from build123d import *

# Parameters (mm, degrees)
SKETCH_1_W          = 66
SKETCH_1_H          = 80.5
EXTRUDE_1_DEPTH     = 5
SKETCH_2_R          = 2
CUT_EXTRUDE_1_DEPTH = 53.288263501
SKETCH_3_R          = 2.1
CUT_EXTRUDE_2_DEPTH = 10
FILLET_1_R          = 15


with BuildPart() as part:
    # 草图1 → 凸台-拉伸1 (new body)
    with BuildSketch(Plane.XY):
        Rectangle(SKETCH_1_W, SKETCH_1_H)
    extrude(amount=EXTRUDE_1_DEPTH)

    # 草图2 → 切除-拉伸1 (cut, through all)
    with BuildSketch(Plane.XY.offset(5)):
        with Locations((-26, 35.25)):
            Circle(SKETCH_2_R)
        with Locations((26, 35.25)):
            Circle(SKETCH_2_R)
        with Locations((26, 25.25)):
            Circle(SKETCH_2_R)
        with Locations((-26, 25.25)):
            Circle(SKETCH_2_R)
    extrude(amount=-CUT_EXTRUDE_1_DEPTH, mode=Mode.SUBTRACT)

    # 草图3 → 切除-拉伸2 (cut)
    with BuildSketch(Plane.XY.offset(5)):
        with Locations((-11, 0.25)):
            Circle(SKETCH_3_R)
        with Locations((11, 0.25)):
            Circle(SKETCH_3_R)
        with Locations((11, -19.75)):
            Circle(SKETCH_3_R)
        with Locations((-11, -19.75)):
            Circle(SKETCH_3_R)
    extrude(amount=-CUT_EXTRUDE_2_DEPTH, mode=Mode.SUBTRACT)

    # 圆角1
    fillet_1_edges = [part.edges().sort_by_distance(p)[0] for p in [
        (33, -40.25, 2.5),
        (-33, -40.25, 2.5),
    ]]
    fillet(fillet_1_edges, radius=FILLET_1_R)


solid = part.part
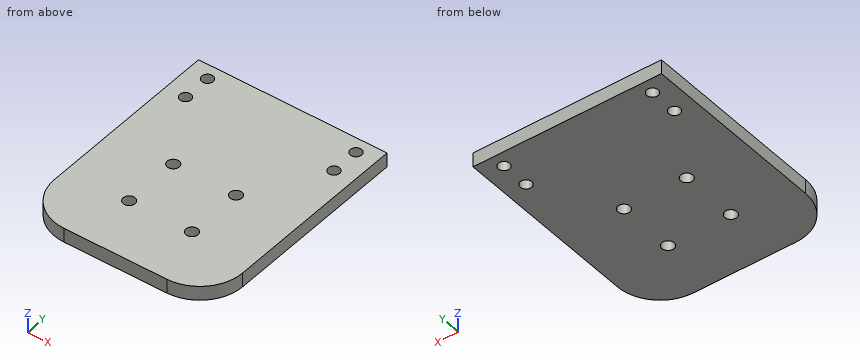
The model under review builds one solid part; all positions refer to its coordinate system, in mm. Round coordinates to 2 decimals unless told otherwise and drop trailing zeros. Write each loop counter-clockwise with the first axis right and the second up, starting at its lowest first coordinate (ties: lowest second). Pieces come first, ordered by that corner, then holes. Notation, with made-up numbers: M 4,82 L 25,82 A17 cw 25,87 Z; hole C 25,-0.75 d2. An arc over 180 degrees is marked long. Answer as CSV lines item,"result". Start each with the question number.
Q1. Consider section A-A, the plane y = 35.25. Give the boundary of the cut face in (x, z), then the cut area to 3 significant figures.
Q2. Consider section B-B, the plane x = -11. Give the boundary of the cut face in (y, z), then the cut area to 4 significant figures.
Q3. Consider section C-C, the plane z = 1.4. State how many separate pieces and enclosed holes the cut face has, then the cut area to 3 significant figures.
Q4. Wall thickness on line 1 along Y through (x, z) = (11, 2.45); line 2 along Y through (x, z) = (26, 1.35); line 3 along Y through (x, z) = (18.5, 1.75): over which ranges is each line inside the solid? List them lowest first.
Q5. Clearance check with a flat-ended pin moving along its axis: P1, Ø2.5, axis at x = 26, y = 25.25, coming from the -Z side. State where the tip first meets the part, or that it passes through.
Result set:
1,outline,"M -33,0 L -28,0 L -28,5 L -33,5 Z; M -24,0 L 24,0 L 24,5 L -24,5 Z; M 28,0 L 33,0 L 33,5 L 28,5 Z"
1,area,"290 mm²"
2,outline,"M -40.25,0 L -21.85,0 L -21.85,5 L -40.25,5 Z; M -17.65,0 L -1.85,0 L -1.85,5 L -17.65,5 Z; M 2.35,0 L 40.25,0 L 40.25,5 L 2.35,5 Z"
2,area,"360.5 mm²"
3,separate pieces,"1"
3,enclosed holes,"8"
3,area,"5,110 mm²"
4,line 1,"y = -40.25 to -21.85, -17.65 to -1.85, 2.35 to 40.25"
4,line 2,"y = -37.94 to 23.25, 27.25 to 33.25, 37.25 to 40.25"
4,line 3,"y = -40.24 to 40.25"
5,P1,"passes through"
